Check sheet for the modelled part. Datum: model origin and axes. Units: mm. A direction names the side the tool comes from. Coordinates: 2 decimals unless noted, no trailing zeros. Write each loop counter-clockwise with the first axis right and the second up, starting at its lowest first coordinate (ties: lowest second). Pieces come first, ordered by that corner, then holes. Notation, with made-up numbers: M -23.75,87.5 L 29.25,87.5 A14 ccw 29.25,112.5 Z; hole C 61.25,-27 d8. An arc over 180 degrees is marked long. Answer as CSV lines item,"result". Start each with the question number.
Q1. Sectioned sample at C-C, the plane x = 10. Record the cut outline in (y, z), then the cut area to 3 significant figures.
Q2. Depth check by flat-ended pin: pin 1 Ø2.5 at (x, y) = (11, 10) entering from +Z. Enter the tip coordinate at first touch or a pass-through.
Q3. Sectioned sample at A-A, the plane z = 14.5. Record the cut outline in (x, y).
Q4. Thickness scan on line 1 along Y through (x, z) = (10, 15.25); line 2 along X through (y, z) = (10.5, 14); line 3 along Z through (x, y) = (8, 10). Record the ranges inside material, lowest first. Write a range as from..to.
Q5. Sectioned sample at B-B, the plane y = 10. Record the cut outline in (x, z), then the cut area to 3 significant figures.
Q6. Access from +Z, -Z, +X, -X, +Y, -Y to the whole of each face (thin tool, end or side, straight path). Record for faces 4 (the flat face through (10, 10, 8)), 5 (the flat face through (40, 10, 0)).
Q7. Mould release check, pull along X, two halves, no side actions. Record for faces 1 (the cylindrical face through (9.46, 7.56, 13.07)), 2 (the flat face through (20, 0, 0)), 3 (the flat face through (0, 10, 0)): pulls with the +X half, pulls with the -X half, needs draft (parallel to the pull), parting line crosses it, or undercut.
from build123d import *

# Parameters (mm, degrees)
ESQUISSE1_W             = 40
ESQUISSE1_H             = 20
BOSS_EXTRU_1_DEPTH      = 18
ESQUISSE2_R             = 2.5
ENL_V_MAT_EXTRU_1_DEPTH = 10


with BuildPart() as part:
    # Esquisse1 → Boss.-Extru.1 (new, symmetric)
    with BuildSketch(Plane.XY):
        with Locations((20, 10)):
            Rectangle(ESQUISSE1_W, ESQUISSE1_H)
    extrude(amount=BOSS_EXTRU_1_DEPTH, both=True)

    # Esquisse2 → Enlèv. mat.-Extru.1 (cut)
    with BuildSketch(Plane.XY.offset(18)):
        with Locations((10, 10)):
            Circle(ESQUISSE2_R)
    extrude(amount=-ENL_V_MAT_EXTRU_1_DEPTH, mode=Mode.SUBTRACT)


solid = part.part
Output:
1,outline,"M 0,-18 L 20,-18 L 20,18 L 12.5,18 L 12.5,8 L 7.5,8 L 7.5,18 L 0,18 Z"
1,area,"670 mm^2"
2,pin 1,"stops at z = 8"
3,outline,"M 0,0 L 40,0 L 40,20 L 0,20 Z; hole C 10,10 d5"
4,line 1,"y = 0..7.5, 12.5..20"
4,line 2,"x = 0..7.55, 12.45..40"
4,line 3,"z = -18..8"
5,outline,"M 0,-18 L 40,-18 L 40,18 L 12.5,18 L 12.5,8 L 7.5,8 L 7.5,18 L 0,18 Z"
5,area,"1,390 mm^2"
6,face 4,"+Z"
6,face 5,"+Z, -Z, +X, +Y, -Y"
7,face 1,"undercut"
7,face 2,"needs draft"
7,face 3,"pulls with the -X half"
